The listing builds one solid part. Answer for the finished solid, in the listing's coordinates (mm). Face numbers are marked on the shaded views. Coordinates: 2 decimals unless noted, no trailing zeros. Loops run counter-clockwise (first coordinate to the right, second up) from the corner with the lowest first, then second, coordinate; pieces in that order, holes last. Notation, with made-up numbers: M 4.5,47.25 L 26.5,47.25 A38 ccw 26.5,85.25 Z; hole C -35.75,-18 d9. An arc over 180 degrees is marked long. Answer in a Markdown table with one row per item. Add a question column.
from build123d import *

# Parameters (mm, degrees)
SKETCH1_R               = 16.7005
SKETCH1_R_2             = 13.0683
BOSS_EXTRUDE1_DEPTH     = 254
CUT_EXTRUDE2_DEPTH      = 256.095694594
CUT_EXTRUDE2_DEPTH_BACK = 256.095694594
SKETCH3_R               = 3.2639
CUT_EXTRUDE3_DEPTH      = 256.095694707
CUT_EXTRUDE3_DEPTH_BACK = 256.095694707
SKETCH4_R               = 3.2639


with BuildPart() as part:
    # Sketch1 → Boss-Extrude1 (new body)
    with BuildSketch(Plane(origin=(0, 0, 0), x_dir=(0, 0, -1), z_dir=(1, 0, 0))):
        Circle(SKETCH1_R)
        Circle(SKETCH1_R_2, mode=Mode.SUBTRACT)
    extrude(amount=BOSS_EXTRUDE1_DEPTH)

    # Sketch3 → Cut-Extrude2 (cut, two sides: drawn at the far end of the back side and taken through both)
    with BuildSketch(Plane(origin=(0, 0, 0), x_dir=(1, 0, 0), z_dir=(0, 1, 0)).offset(-CUT_EXTRUDE2_DEPTH_BACK)):
        with Locations(Location((127, 0, 0), (0, 0, 270))):
            Circle(SKETCH3_R)
    extrude(amount=CUT_EXTRUDE2_DEPTH + CUT_EXTRUDE2_DEPTH_BACK, mode=Mode.SUBTRACT)

    # Sketch4 → Cut-Extrude3 (cut, two sides: drawn at the far end of the back side and taken through both)
    with BuildSketch(Plane(origin=(0, 0, 0), x_dir=(-1, 0, 0), z_dir=(0, 0.819152044288991, -0.5735764363510473)).offset(-CUT_EXTRUDE3_DEPTH_BACK)):
        with Locations(Location((-203.2, 0, 0), (0, 0, 90))):
            Circle(SKETCH4_R)
        with Locations(Location((-50.8, 0, 0), (0, 0, 90))):
            Circle(SKETCH4_R)
    extrude(amount=CUT_EXTRUDE3_DEPTH + CUT_EXTRUDE3_DEPTH_BACK, mode=Mode.SUBTRACT)


solid = part.part
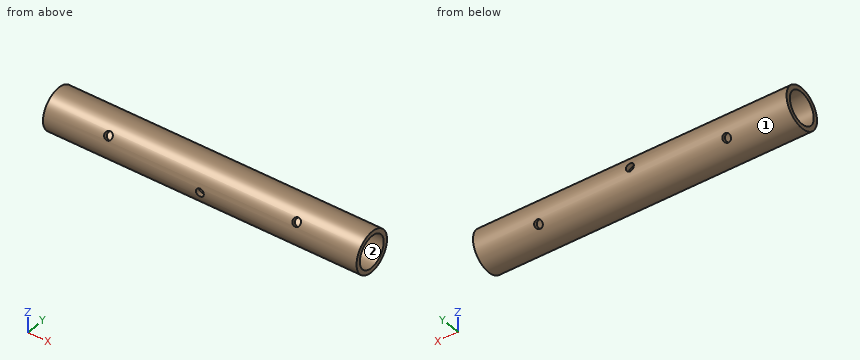
(1) A cutting plane is placed at D-D (x = 234). Give the vertices of the cut face in (y, z).
(2) Straight lines are drawn through the part: line 1 (Y direction, x = 171, z = 0); line 2 (X direction, y = 15.45, z = 0); line 3 (Y direction, x = 129, z = -9.5). For each, find the intervals that lie inside material, in ascending order.
(3) A cutting plane is placed at B-B (y = 0). Give the vertices of the cut face in (x, z), plus the area to 3 significant figures.
(4) The mould has two halves that part along Z. Classify the marked faces 1 and 2: released by +Z, released by -Z, zero draft, split by the parting line, or undercut.
(5) Each of these flat-tipped pins is pushed along its axis until it touches: pin 1 (6 mm diameter, centred on x = 127, z = 0, fed in from +Y); pin 2 (12 mm diameter, centred on x = 47.5, y = -9, fed in from -Z); pin 3 (6 mm diameter, centred on x = 167.5, y = -5.5, fed in from +Z); pin 4 (4 mm diameter, centred on x = 107, y = -11, fed in from +Z). Where does it stop, or does it pass through?
(6) A cutting plane is placed at A-A (z = 0). Give the vertices of the cut face in (x, y), plus the area to 3 significant figures.
(7) A cutting plane is placed at C-C (x = 127). Give the vertices of the cut face in (y, z), plus the area to 3 significant figures.
Solved:
| question | item | result |
|---|---|---|
| 1 | outline | C 0,0 d33.4; hole C 0,0 d26.14 |
| 2 | line 1 | y = -16.7 to -13.07, 13.07 to 16.7 |
| 2 | line 2 | x = 0 to 123.74, 130.26 to 254 |
| 2 | line 3 | y = -13.74 to -8.97, 8.97 to 13.74 |
| 3 | outline | M 0,-16.7 L 254,-16.7 L 254,-13.07 L 0,-13.07 Z; M 0,13.07 L 254,13.07 L 254,16.7 L 0,16.7 Z |
| 3 | area | 1,850 mm² |
| 4 | face 1 | split by the parting line |
| 4 | face 2 | undercut |
| 5 | pin 1 | passes through |
| 5 | pin 2 | stops at z = -16.43 |
| 5 | pin 3 | stops at z = 16.51 |
| 5 | pin 4 | stops at z = 14.07 |
| 6 | outline | M 0,-16.7 L 123.74,-16.7 L 123.74,-13.07 L 0,-13.07 Z; M 0,13.07 L 123.74,13.07 L 123.74,16.7 L 0,16.7 Z; M 130.26,-16.7 L 254,-16.7 L 254,-13.07 L 130.26,-13.07 Z; M 130.26,13.07 L 254,13.07 L 254,16.7 L 130.26,16.7 Z |
| 6 | area | 1,800 mm² |
| 7 | outline | M -16.38,-3.26 A16.7 ccw 16.38,-3.26 L 12.65,-3.26 A13.07 cw -12.65,-3.26 Z; M -16.38,3.26 L -12.65,3.26 A13.07 cw 12.65,3.26 L 16.38,3.26 A16.7 ccw Z |
| 7 | area | 292 mm² |
